from build123d import *

# Parameters (mm, degrees)
F0_R      = 9.525
F1_DEPTH  = 9.525
F2_R      = 12.7
F2_R_2    = 9.525
F3_DEPTH  = 3.175
F5_DEPTH  = 25.4
F6_R      = 3.7846
F6_R_2    = 3.048
F7_DEPTH  = 6.604
F7_FACE_R = 3.048
F8_DEPTH  = 12.701
F10_DEPTH = 2.286


with BuildPart() as f1:
    # F0 (on Top) → F1 (new body)
    with BuildSketch(Plane.XY):
        Circle(F0_R)
    extrude(amount=F1_DEPTH)

    # F2 (on face) → F3 (join)
    with BuildSketch(Plane.XY.offset(9.525)):
        Circle(F2_R)
        Circle(F2_R_2, mode=Mode.SUBTRACT)
        Circle(F2_R_2)
    extrude(amount=F3_DEPTH)

    # F4 (on face) → F5 (cut)
    with BuildSketch(Plane.XY.offset(12.7)):
        with BuildLine():
            ThreePointArc((-9.525, 8.40026), (-12.7, 0), (-9.525, -8.40026))
            Line((-9.525, -8.40026), (-9.525, 8.40026))
        make_face()
        with BuildLine():
            Line((9.525, 8.40026), (9.525, -8.40026))
            ThreePointArc((9.525, -8.40026), (11.879762, -4.490128), (12.7, 0))
            ThreePointArc((12.7, 0), (11.879762, 4.490128), (9.525, 8.40026))
        make_face()
    extrude(amount=-F5_DEPTH, mode=Mode.SUBTRACT)

    # F6 (on face) → F7 (join)
    with BuildSketch(Plane.XY.offset(12.7)):
        Circle(F6_R)
        Circle(F6_R_2, mode=Mode.SUBTRACT)
    extrude(amount=F7_DEPTH)

    # F7_face (on face) → F8 (cut, through all)
    with BuildSketch(Plane.XY.offset(12.7)):
        Circle(F7_FACE_R)
    extrude(amount=-F8_DEPTH, mode=Mode.SUBTRACT)

    # F9 (on face) → F10 (cut)
    with BuildSketch(Plane.XY.offset(19.304)):
        with BuildLine():
            Line((3.741201, -0.5715), (4.079275, -0.5715))
            Line((4.079275, -0.5715), (4.079275, 0.5715))
            Line((4.079275, 0.5715), (3.741201, 0.5715))
            ThreePointArc((3.741201, 0.5715), (3.773735, 0.286573), (3.7846, 0))
            ThreePointArc((3.7846, 0), (3.773735, -0.286573), (3.741201, -0.5715))
        make_face()
        with BuildLine():
            Line((-4.079275, -0.5715), (-3.741201, -0.5715))
            ThreePointArc((-3.741201, -0.5715), (-3.7846, 0), (-3.741201, 0.5715))
            Line((-3.741201, 0.5715), (-4.079275, 0.5715))
            Line((-4.079275, 0.5715), (-4.079275, -0.5715))
        make_face()
        with BuildLine():
            ThreePointArc((-3.741201, 0.5715), (-3.7846, 0), (-3.741201, -0.5715))
            Line((-3.741201, -0.5715), (-2.993943, -0.5715))
            ThreePointArc((-2.993943, -0.5715), (-3.048, 0), (-2.993943, 0.5715))
            Line((-2.993943, 0.5715), (-3.741201, 0.5715))
        make_face()
        with BuildLine():
            Line((2.993943, -0.5715), (3.741201, -0.5715))
            ThreePointArc((3.741201, -0.5715), (3.773735, -0.286573), (3.7846, 0))
            ThreePointArc((3.7846, 0), (3.773735, 0.286573), (3.741201, 0.5715))
            Line((3.741201, 0.5715), (2.993943, 0.5715))
            ThreePointArc((2.993943, 0.5715), (3.034456, 0.287025), (3.048, 0))
            ThreePointArc((3.048, 0), (3.034456, -0.287025), (2.993943, -0.5715))
        make_face()
        with BuildLine():
            Line((-2.993943, -0.5715), (2.993943, -0.5715))
            ThreePointArc((2.993943, -0.5715), (3.034456, -0.287025), (3.048, 0))
            ThreePointArc((3.048, 0), (3.034456, 0.287025), (2.993943, 0.5715))
            Line((2.993943, 0.5715), (-2.993943, 0.5715))
            ThreePointArc((-2.993943, 0.5715), (-3.048, 0), (-2.993943, -0.5715))
        make_face()
    extrude(amount=-F10_DEPTH, mode=Mode.SUBTRACT)


solid = f1.part
Read the model definition and answer for the solid it produces. Units are mm, in the model's axes. A direction names the side the tool comes from. Round coordinates to 2 decimals unless told otherwise and drop trailing zeros. Order: outer loops, then holes, each group sorted by start corner. A loop starts at its lowest first (then second) coordinate and runs counter-clockwise, first axis right, second up. Notation, with made-up numbers: (-29.75, 68) - (-10.75, 68) arc R20 ccw to (-10.75, 104) - close; hole circle Ø4 at (-16.5, 23). An arc over 180 degrees is marked (long way). Use one line per item in the form item = value. Start each with the question number.
(1) The part is cut by section C-C (z = 10). Give the vertices of the cut face in (x, y) (3 decimals).
(2) Determine the mould class of faces 6 (the face through (0, 10, 9.525)), 7 (the face through (3.61, 1.14, 15.96)), 8 (the face through (2.907, 0.916, 9.787)), 9 (the face through (-0.2, -12.7, 11.1)) for opening direction Y: +Y half, -Y half, draft (parallel to the pull), parting line (faces both ways), or undercut.
(3) Flat-ended cylindrical pins translate along their axes: pin 1 Ø2 at (x, z) = (6, 2) entering from -Y; pin 2 Ø0.6 at (x, z) = (-3.5, 18.5) entering from +Y; pin 3 Ø3 at (x, z) = (2, 3) entering from +Y; pin 4 Ø5 at (x, y) = (-5, 2.5) entering from -Z. Find the tip coordinate at first contact, or state that the pin passes through.
(4) The part is cut by section D-D (y = 4.75). Give the vertices of the cut face in (x, z) (3 decimals), then the cut area to 3 significant figures.
(5) Find the intervals of material crossed by line 1 along X through (y, z) = (0, 14); line 2 along Y through (x, z) = (0, 12); line 3 along Y through (x, z) = (0, 5) (3 decimals), in increasing order. Write a range as from..to.
(6) For faces 1 (the face through (-7.559, -5.796, 4.696)), 2 (the face through (0.3, 3.3, 19.304)), 3 (the face through (-9.525, 0, 11)), 4 (the face through (-1, -10, 9.525)), 5 (the face through (-4, 0, 12.7)), determine the directions among +Z, -Z, +X, -X, +Y, -Y from which every point of the face is accessible in a straight line to the end or side of a thin tool.
(7) The part is cut by section A-A (x = 0). Give the vertices of the cut face in (y, z) (3 decimals), then the cut area to 3 significant figures.
Checked values:
q1.outline = (-9.525, -8.4) arc R12.7 ccw to (9.525, -8.4) - (9.525, 8.4) arc R12.7 ccw to (-9.525, 8.4) - close; hole circle Ø6.096 at (0, 0)
q2.face_6 = draft
q2.face_7 = parting line
q2.face_8 = undercut
q2.face_9 = -Y half
q3.pin_1 = -8.11
q3.pin_2 = 2.02
q3.pin_3 = 9.51
q3.pin_4 = 0
q4.outline = (-9.525, 9.525) - (-8.256, 9.525) - (-8.256, 0) - (8.256, 0) - (8.256, 9.525) - (9.525, 9.525) - (9.525, 12.7) - (-9.525, 12.7) - close
q4.area = 218 mm^2
q5.line_1 = -3.78..-3.05, 3.05..3.78
q5.line_2 = -12.7..-3.05, 3.05..12.7
q5.line_3 = -9.525..-3.048, 3.048..9.525
q6.face_1 = -Z
q6.face_2 = +Z, +X, -X, +Y, -Y
q6.face_3 = +Z, -Z, -X, +Y, -Y
q6.face_4 = -Z, -Y
q6.face_5 = +Z
q7.outline = (-12.7, 9.525) - (-9.525, 9.525) - (-9.525, 0) - (-3.048, 0) - (-3.048, 19.304) - (-3.785, 19.304) - (-3.785, 12.7) - (-12.7, 12.7) - close; (3.048, 0) - (9.525, 0) - (9.525, 9.525) - (12.7, 9.525) - (12.7, 12.7) - (3.785, 12.7) - (3.785, 19.304) - (3.048, 19.304) - close
q7.area = 194 mm^2
